Here's how the part is built. I have some questions about the finished solid (model axes, mm). A direction names the side the tool comes from. Round coordinates to 2 decimals unless told otherwise and drop trailing zeros. Loops run counter-clockwise (first coordinate to the right, second up) from the corner with the lowest first, then second, coordinate; pieces in that order, holes last. Notation, with made-up numbers: M 34,3 L 56,3 A9 ccw 56,13 Z; hole C 7.25,22 d11. An arc over 180 degrees is marked long. Use a Markdown table: item, result.
from build123d import *

# Parameters (mm, degrees)
SKETCH3_R           = 10
SKETCH3_R_2         = 7
BASE_DEPTH          = 5
SKETCH3_2_R         = 7
BOSS_EXTRUDE4_DEPTH = 14.24
SKETCH4_R           = 3.3
SKETCH4_R_2         = 1.65
CUT_EXTRUDE4_DEPTH  = 5
CUT_EXTRUDE5_START  = -9.99
SKETCH4_3_R         = 5
SKETCH4_3_R_2       = 3.3
SKETCH4_3_R_3       = 1.65
CUT_EXTRUDE5_DEPTH  = 4.25
SKETCH4_4_R         = 1.65
CUT_EXTRUDE6_DEPTH  = 21.069319869
F_2_MOVE_FACE1_BY   = 0.2
F_2_MOVE_FACE1_2_BY = 0.2
F_2_MOVE_FACE1_3_BY = 0.2
F_2_MOVE_FACE1_4_BY = 0.2
CHAMFER1_SIZE       = 0.5
CHAMFER2_SIZE       = 1


with BuildPart() as part:
    # Sketch3 → Base (new body)
    with BuildSketch(Plane(origin=(0, 0, 0), x_dir=(1, 0, 0), z_dir=(0, 1, 0))):
        with Locations(Location((0, 0, 0), (0, 0, 270))):
            Circle(SKETCH3_R)
        with Locations(Location((0, 0, 0), (0, 0, 270))):
            Circle(SKETCH3_R_2, mode=Mode.SUBTRACT)
    extrude(amount=-BASE_DEPTH)

    # Sketch3<2> → Boss-Extrude4 (add)
    with BuildSketch(Plane(origin=(0, 0, 0), x_dir=(1, 0, 0), z_dir=(0, 1, 0))):
        with Locations(Location((0, 0, 0), (0, 0, 270))):
            Circle(SKETCH3_2_R)
    extrude(amount=-BOSS_EXTRUDE4_DEPTH)

    # Sketch4 → Cut-Extrude4 (cut)
    with BuildSketch(Plane(origin=(0, 0, 0), x_dir=(1, 0, 0), z_dir=(0, 1, 0))):
        with Locations(Location((0, 0, 0), (0, 0, 270))):
            Circle(SKETCH4_R)
        with Locations(Location((0, 0, 0), (0, 0, 270))):
            Circle(SKETCH4_R_2, mode=Mode.SUBTRACT)
    extrude(amount=-CUT_EXTRUDE4_DEPTH, mode=Mode.SUBTRACT)

    # Sketch4<3> → Cut-Extrude5 (cut)
    # profile 1 of 3: a face of its own
    with BuildSketch(Plane(origin=(0, 0, 0), x_dir=(1, 0, 0), z_dir=(0, 1, 0)).offset(CUT_EXTRUDE5_START)):
        with Locations(Location((0, 0, 0), (0, 0, 270))):
            Circle(SKETCH4_3_R)
        with Locations(Location((0, 0, 0), (0, 0, 270))):
            Circle(SKETCH4_3_R_2, mode=Mode.SUBTRACT)
    # profile 2 of 3: a face of its own
    with BuildSketch(Plane(origin=(0, 0, 0), x_dir=(1, 0, 0), z_dir=(0, 1, 0)).offset(CUT_EXTRUDE5_START)):
        with Locations(Location((0, 0, 0), (0, 0, 270))):
            Circle(SKETCH4_3_R_2)
        with Locations(Location((0, 0, 0), (0, 0, 270))):
            Circle(SKETCH4_3_R_3, mode=Mode.SUBTRACT)
    # profile 3 of 3: a face of its own
    with BuildSketch(Plane(origin=(0, 0, 0), x_dir=(1, 0, 0), z_dir=(0, 1, 0)).offset(CUT_EXTRUDE5_START)):
        with Locations(Location((0, 0, 0), (0, 0, 270))):
            Circle(SKETCH4_3_R_3)
    extrude(amount=-CUT_EXTRUDE5_DEPTH, mode=Mode.SUBTRACT)

    # Sketch4<4> → Cut-Extrude6 (cut, through all)
    with BuildSketch(Plane(origin=(0, 0, 0), x_dir=(1, 0, 0), z_dir=(0, 1, 0))):
        with Locations(Location((0, 0, 0), (0, 0, 270))):
            Circle(SKETCH4_4_R)
    extrude(amount=-CUT_EXTRUDE6_DEPTH, mode=Mode.SUBTRACT)

    # .2 Move Face1: a curved face moved inward by 0.2
    add(Solid.thicken(part.faces().sort_by_distance((0, -12.115, -5))[0], -F_2_MOVE_FACE1_BY), mode=Mode.SUBTRACT)

    # 2 Move Face1 2: a curved face moved inward by 0.2
    add(Solid.thicken(part.faces().sort_by_distance((0, -7.495, -1.65))[0], -F_2_MOVE_FACE1_2_BY), mode=Mode.SUBTRACT)

    # 2 Move Face1 3: a face moved inward by 0.2
    extrude(part.faces().sort_by_distance((0, -5, 2.64))[0], amount=F_2_MOVE_FACE1_3_BY, dir=(0, -1, 0), mode=Mode.SUBTRACT)

    # 2 Move Face1 4: a curved face moved inward by 0.2
    add(Solid.thicken(part.faces().sort_by_distance((0, -2.5, -3.3))[0], -F_2_MOVE_FACE1_4_BY), mode=Mode.SUBTRACT)

    # Chamfer1
    chamfer1_edges = [part.edges().sort_by_distance(p)[0] for p in [
        (0, -14.24, -7),
        (0, -14.24, -5.2),
    ]]
    chamfer(chamfer1_edges, length=CHAMFER1_SIZE)

    # Chamfer2
    chamfer2_edges = [part.edges().sort_by_distance(p)[0] for p in [
        (0, -5, -10),
    ]]
    chamfer(chamfer2_edges, length=CHAMFER2_SIZE)


solid = part.part
1. Imagine slicing it at A-A, the plane x = 0. Write out the boundary of the cut face in (y, z).
Answer sheet:
| item | result |
|---|---|
| outline | M -14.24,-6.5 L -13.74,-7 L -5,-7 L -5,-9 L -4,-10 L 0,-10 L 0,-3.5 L -5.2,-3.5 L -5.2,-1.85 L -9.99,-1.85 L -9.99,-5.2 L -13.74,-5.2 L -14.24,-5.7 Z; M -14.24,5.7 L -13.74,5.2 L -9.99,5.2 L -9.99,1.85 L -5.2,1.85 L -5.2,3.5 L 0,3.5 L 0,10 L -4,10 L -5,9 L -5,7 L -13.74,7 L -14.24,6.5 Z |
2. We'd pull the mould along X, two halves only. Please class faces 1 (the face through (-6.834, -9.309, -1.517)), 2 (the face through (-2, -5.2, 2)), 3 (the face through (-3.417, -2.564, -0.759)), 4 (the face through (-6, -14.24, 0)): +X half, -X half, draft (parallel to the pull), parting line (faces both ways), or undercut.
Answer sheet:
| item | result |
|---|---|
| face 1 | parting line |
| face 2 | undercut |
| face 3 | undercut |
| face 4 | draft |
3. I need wall thicknesses on probe 1 along X at (y, z) = (-7.5, 0); probe 2 along X at (y, z) = (-12, 0); probe 3 along Z at (x, y) = (1.25, -12.25). Which ranges of each line are inside material? Lowest first, please. Write a range as from..to.
Answer sheet:
| item | result |
|---|---|
| probe 1 | -7..-1.85, 1.85..7 |
| probe 2 | -7..-5.2, 5.2..7 |
| probe 3 | -6.89..-5.05, 5.05..6.89 |
4. Which directions (+Z, -Z, +X, -X, +Y, -Y) give clear straight access to the entire face, cutting with the end or side of a thin tool? Please do faces 5 (the face through (1.56, -11.84, 4.96)), 6 (the face through (-9.76, -1.97, -2.17)).
Answer sheet:
| item | result |
|---|---|
| face 5 | -Y |
| face 6 | +Y, -Y |
5. Imagine slicing it at D-D, the plane y = -8. Write out the boundary of the cut face in (x, z).
Answer sheet:
| item | result |
|---|---|
| outline | C 0,0 d14; hole C 0,0 d3.7 |
6. Imagine slicing it at B-B, the plane z = 0. Write out the boundary of the cut face in (x, y).
Answer sheet:
| item | result |
|---|---|
| outline | M -10,-4 L -9,-5 L -7,-5 L -7,-13.74 L -6.5,-14.24 L -5.7,-14.24 L -5.2,-13.74 L -5.2,-9.99 L -1.85,-9.99 L -1.85,-5.2 L -3.5,-5.2 L -3.5,0 L -10,0 Z; M 1.85,-9.99 L 5.2,-9.99 L 5.2,-13.74 L 5.7,-14.24 L 6.5,-14.24 L 7,-13.74 L 7,-5 L 9,-5 L 10,-4 L 10,0 L 3.5,0 L 3.5,-5.2 L 1.85,-5.2 Z |
7. Imagine slicing it at C-C, the plane y = -10.5. Write out the boundary of the cut face in (x, z).
Answer sheet:
| item | result |
|---|---|
| outline | C 0,0 d14; hole C 0,0 d10.4 |
8. For pin 1 Ø3 at (y, z) = (-5.5, -6.5) entering from -X; pin 2 Ø11 at (x, z) = (0, 0) entering from -Y; pin 3 Ø8 at (x, y) = (-5.5, -12.5) entering from -Z, each with a flat end and sliding along its axis, tell me the tip position at first contact or that it passes through.
Answer sheet:
| item | result |
|---|---|
| pin 1 | x = -7.93 |
| pin 2 | y = -14.04 |
| pin 3 | z = -6.84 |
